from build123d import *

# Parameters (mm, degrees)
F0_W           = 40
F0_H           = 40
F1_DEPTH       = 6
F4_D           = 3.4
F4_CBORE_D     = 5.5
F4_CBORE_DEPTH = 3
F5_D           = 3.4
F6_DEPTH       = 2.5


with BuildPart() as f1:
    # F0 (on Top) → F1 (new body)
    with BuildSketch(Plane.XY):
        Rectangle(F0_W, F0_H)
    extrude(amount=F1_DEPTH)

    # F4 (through all)
    with Locations(Plane.XY.offset(6)):
        with Locations((-15.5, 15.5), (15.5, 15.5), (15.5, -15.5), (-15.5, -15.5)):
            CounterBoreHole(F4_D / 2, F4_CBORE_D / 2, F4_CBORE_DEPTH)

    # F5 (through all)
    with Locations(Plane(origin=(0, 0, 0), x_dir=(1, 0, 0), z_dir=(0, 0, -1))):
        with Locations((-11.5, -11.5), (11.5, -11.5), (11.5, 11.5), (-11.5, 11.5)):
            Hole(F5_D / 2)

    # F3 (on face) → F6 (cut)
    with BuildSketch(Plane.XY):
        Polygon((-9.8625, 8.663767), (-8.225, 11.5), (-9.8625, 14.336233), (-13.1375, 14.336233), (-14.775, 11.5), (-13.1375, 8.663767), align=None)
        Polygon((-9.8625, -14.336233), (-8.225, -11.5), (-9.8625, -8.663767), (-13.1375, -8.663767), (-14.775, -11.5), (-13.1375, -14.336233), align=None)
        Polygon((8.225, -11.5), (9.8625, -14.336233), (13.1375, -14.336233), (14.775, -11.5), (13.1375, -8.663767), (9.8625, -8.663767), align=None)
        Polygon((8.225, 11.5), (9.8625, 8.663767), (13.1375, 8.663767), (14.775, 11.5), (13.1375, 14.336233), (9.8625, 14.336233), align=None)
    extrude(amount=F6_DEPTH, mode=Mode.SUBTRACT)


solid = f1.part
Part model, mm, in its own coordinate system. A direction names the side the tool comes from. Round coordinates to 2 decimals unless told otherwise and drop trailing zeros. Write each loop counter-clockwise with the first axis right and the second up, starting at its lowest first coordinate (ties: lowest second). Pieces come first, ordered by that corner, then holes. Notation, with made-up numbers: M 51,60 L 65,60 A26 ccw 65,74 Z; hole C -32,2 d7. An arc over 180 degrees is marked long. Return JSON: item names as keys, results as strings. Group by question number.
(1) Two-plate mould, pull along X, no slides. Class faces 4 (the face through (0, 0, 0)), 5 (the face through (13.945, 10.062, 1.232)), 6 (the face through (20, 0, 3)): +X half, -X half, draft (parallel to the pull), parting line (faces both ways), or undercut.
(2) Drill centre lines: probe 1 along Y at (x, z) = (13, 2.4); probe 2 along Y at (x, z) = (15.5, 5.15); probe 3 along X at (y, z) = (-11.5, 4.65). Where is each one in solid material? Low to high.
(3) Which spindle directions (+Z, -Z, +X, -X, +Y, -Y) get a long thin tool onto all of the face, cutting with end or side? Do faces 1 (the face through (-14, 17, 3)), 2 (the face through (13.945, -12.938, 1.232)), 3 (the face through (-12.3, 13, 4.3)). Say none if no direction does.
(4) Saw through at A-A on x = 15.5. Write the cut outline in (y, z).
(5) Pin check, flat tips, straight feed: pin 1 Ø1.7 at (x, y) = (10, 12) entering from -Z; pin 2 Ø3.5 at (x, y) = (-15.5, 15.5) entering from +Z. Stop position of each tip, or through.
(6) Saw through at C-C on z = 5.45. Count the separate pieces of the cut face and the enclosed holes in it, then the cut area to 3 significant figures.
Returned:
{
 "1": {"face 4": "draft", "face 5": "undercut", "face 6": "+X half"},
 "2": {"probe 1": "-20 to -14.34, -8.66 to 8.66, 14.34 to 20", "probe 2": "-20 to -18.25, -12.75 to 12.75, 18.25 to 20", "probe 3": "-20 to -13.2, -9.8 to 9.8, 13.2 to 20"},
 "3": {"face 1": "+Z", "face 2": "-Z", "face 3": "+Z, -Z"},
 "4": {"outline": "M -20,0 L -17.2,0 L -17.2,3 L -18.25,3 L -18.25,6 L -20,6 Z; M -13.8,0 L 13.8,0 L 13.8,3 L 12.75,3 L 12.75,6 L -12.75,6 L -12.75,3 L -13.8,3 Z; M 17.2,0 L 20,0 L 20,6 L 18.25,6 L 18.25,3 L 17.2,3 Z"},
 "5": {"pin 1": "z = 2.5", "pin 2": "z = 3"},
 "6": {"separate pieces": "1", "enclosed holes": "8", "area": "1,470 mm²"}
}
